Drawing for the job (mm, zero at the part's lowest x, y, z). A direction names the side the tool comes from. Give positions to 0.01 mm unless a question says otherwise; leave off trailing zeros. Loops run counter-clockwise (first coordinate to the right, second up) from the corner with the lowest first, then second, coordinate; pieces in that order, holes last. Notation, with made-up numbers: (22, 70.5) -> (59, 70.5) arc R21 ccw to (59, 92.5) -> close; hole circle Ø3 at (3, -27.75). An arc over 180 degrees is marked (long way). Write item = value, one per line.
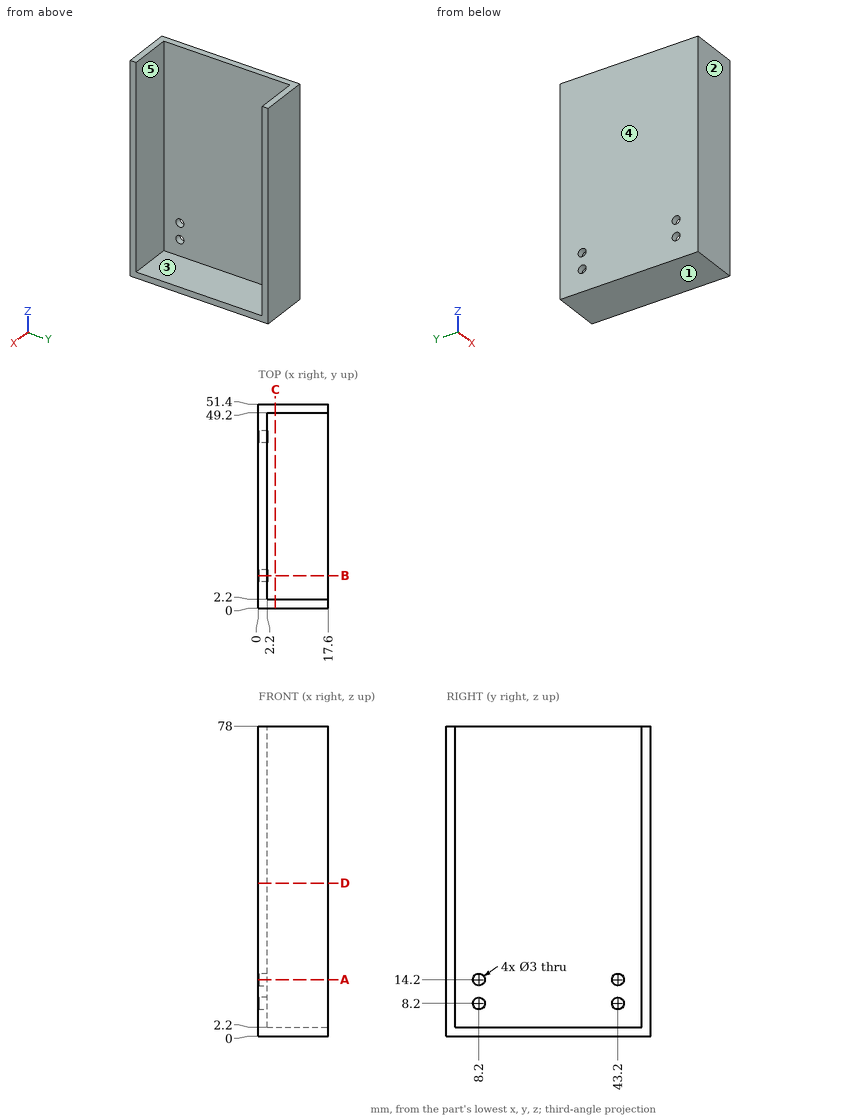
1) Pull direction Y, two halves, no side cores. Call the marked faces 1, 2 and 3: pulls with the +Y half, pulls with the -Y half, needs draft (parallel to the pull), parting line crosses it, or undercut.
Resolved:
face_1 = needs draft
face_2 = pulls with the -Y half
face_3 = undercut
2) Slice it at B-B, the plane y = 8.2. List the corners of the cut face in (x, z).
Resolved:
outline = (0, 0) -> (17.6, 0) -> (17.6, 2.2) -> (2.2, 2.2) -> (2.2, 6.7) -> (0, 6.7) -> close; (0, 9.7) -> (2.2, 9.7) -> (2.2, 12.7) -> (0, 12.7) -> close; (0, 15.7) -> (2.2, 15.7) -> (2.2, 78) -> (0, 78) -> close
3) Slice it at C-C, the plane x = 4.25. List the corners of the cut face in (y, z).
Resolved:
outline = (0, 0) -> (51.4, 0) -> (51.4, 78) -> (49.2, 78) -> (49.2, 2.2) -> (2.2, 2.2) -> (2.2, 78) -> (0, 78) -> close
4) Which spindle directions (+Z, -Z, +X, -X, +Y, -Y) get a long thin tool onto all of the face, cutting with end or side? Do the marked faces 4 and 5. Say none if no direction does.
Resolved:
face_4 = +Z, -Z, -X, +Y, -Y
face_5 = +Z, +X
5) Drop flat-ended pins along their axis: P1, Ø2, axis at x = 14.5, y = 10.5, coming from the +Z side; P2, Ø14, axis at y = 15, z = 33.5, coming from the +X side; P3, Ø1.8, axis at y = 8.2, z = 14.2, coming from the -X side. Give the stop position or say it passes through.
Resolved:
P1 = 2.2
P2 = 2.2
P3 = through
6) Slice it at A-A, the plane z = 14.2. List the corners of the cut face in (x, y), and give its area (3 significant figures).
Resolved:
outline = (0, 0) -> (17.6, 0) -> (17.6, 2.2) -> (2.2, 2.2) -> (2.2, 6.7) -> (0, 6.7) -> close; (0, 9.7) -> (2.2, 9.7) -> (2.2, 41.7) -> (0, 41.7) -> close; (0, 44.7) -> (2.2, 44.7) -> (2.2, 49.2) -> (17.6, 49.2) -> (17.6, 51.4) -> (0, 51.4) -> close
area = 168 mm²
7) Drill centre lines: line 1 along Y through (x, z) = (0.85, 14.2); line 2 along Z through (x, y) = (0.9, 43.2); line 3 along Y through (x, z) = (12.75, 16). Where is each one in solid material? Low to high. Write a range as [from, to].
Resolved:
line_1 = [0, 6.7], [9.7, 41.7], [44.7, 51.4]
line_2 = [0, 6.7], [9.7, 12.7], [15.7, 78]
line_3 = [0, 2.2], [49.2, 51.4]
8) Slice it at D-D, the plane z = 38.5. List the corners of the cut face in (x, y).
Resolved:
outline = (0, 0) -> (17.6, 0) -> (17.6, 2.2) -> (2.2, 2.2) -> (2.2, 49.2) -> (17.6, 49.2) -> (17.6, 51.4) -> (0, 51.4) -> close
